CAD build for the part. Positions are in the model's coordinates, mm. Face numbers are marked on the shaded views. Round coordinates to 2 decimals unless told otherwise and drop trailing zeros. Loops run counter-clockwise (first coordinate to the right, second up) from the corner with the lowest first, then second, coordinate; pieces in that order, holes last. Notation, with made-up numbers: M 39,80 L 50,80 A17 cw 50,97 Z; hole C -34,-36.5 d10. An arc over 180 degrees is marked long. Put each result on its own line as item: value. Start each with the question number.
Autodesk Inventor part; units mm, degrees
ref_plane "YZ Plane" through (0, 0, 0) normal (1, 0, 0) x (0, 1, 0)
ref_plane "XZ Plane" through (0, 0, 0) normal (0, 1, 0) x (-1, 0, 0)
ref_plane "XY Plane" through (0, 0, 0) normal (0, 0, 1) x (1, 0, 0)
sketch "Sketch1" plane through (0, 0, 0) normal (0, 1, 0) x (-1, 0, 0)
  line L0 (0, 0) -> (0, -88.265)
  line L1 (0, -88.265) -> (41.275, -88.265)
  line L2 (0, 0) -> (23.8125, 0)
  line L3 (32.4358, -34.29) -> (32.4358, -59.69)
  line L4 (41.275, -88.265) -> (41.275, -81.915)
  line L5 (23.8125, 0) -> (23.8125, -6.35)
  line L6 (23.8125, -6.35) -> (32.4358, -34.29)
  line L7 (32.4358, -59.69) -> (41.275, -81.915)
  line L8 (33.655, -88.265) -> (33.655, -80.645)
  line L9 (7.62, -88.265) -> (7.62, -80.645)
  line L10 (7.62, -80.645) -> (33.655, -80.645)
  line L11 (16.1925, 0) -> (16.1925, -7.62)
  line L12 (16.1925, -7.62) -> (7.62, -7.62)
  line L13 (7.62, -7.62) -> (7.62, 0)
  point P0 (32.4358, -46.99)
  dimension "d0" = 88.265
  dimension "d1" = 41.275
  dimension "d2" = 23.8125
  dimension "d3" = 41.275
  dimension "d4" = 32.4358
  dimension "d5" = 25.4
  dimension "d6" = 12.7
  dimension "d10" = 6.35
  dimension "d11" = 6.35
  dimension "d12" = 7.62
  dimension "d13" = 7.62
  dimension "d14" = 7.62
  dimension "d15" = 7.62
  dimension "d16" = 7.62
  dimension "d17" = 7.62
extrude "Extrusion1" add sketch "Sketch1" along normal blind 6.985 contours L2 L13 L12 L11 L5 L6 L3 L7 L4 L1 L8 L10 L9 L0
fillet "Fillet2" radius 3.175 12 edges at (-41.275, 3.4925, -81.915) (-32.4358, 3.4925, -59.69) (-32.4358, 3.4925, -34.29) (-23.8125, 3.4925, -6.35) (-3.81, 0, 0) (-3.81, 6.985, 0) (-20.0025, 0, 0) (-20.0025, 6.985, 0) (-37.465, 0, -88.265) (-37.465, 6.985, -88.265) (-3.81, 0, -88.265) (-3.81, 6.985, -88.265)
sketch "Sketch2" plane through (0, 6.985, 0) normal (0, 1, 0) x (1, 0, 0)
  line L0 (-7.62, 85.09) -> (0, 85.09)
  line L1 (-7.62, 85.09) -> (-7.62, 80.645)
  line L2 (-7.62, 80.645) -> (-33.655, 80.645)
  line L3 (-33.655, 80.645) -> (-33.655, 85.09)
  line L4 (-41.275, 85.09) -> (-33.655, 85.09)
  line L5 (-41.275, 85.09) -> (-41.275, 82.5232)
  arc A0 (-41.275, 82.5232) -> (-41.0502, 81.3499) centre (-38.1, 82.5232) ccw
  line L6 (-41.0502, 81.3499) -> (-32.6606, 60.2551)
  arc A1 (-32.4358, 59.0818) -> (-32.6606, 60.2551) centre (-35.6108, 59.0818) ccw
  line L7 (-32.4358, 59.0818) -> (-32.4358, 34.7688)
  arc A2 (-32.4358, 34.7688) -> (-32.2946, 33.8325) centre (-29.2608, 34.7688) ccw
  line L8 (-32.2946, 33.8325) -> (-23.9537, 6.8075)
  arc A3 (-23.8125, 5.8712) -> (-23.9537, 6.8075) centre (-26.9875, 5.8712) ccw
  line L9 (-23.8125, 5.8712) -> (-23.8125, 3.175)
  line L10 (-16.1925, 3.175) -> (-23.8125, 3.175)
  line L11 (-16.1925, 3.175) -> (-16.1925, 7.62)
  line L12 (-16.1925, 7.62) -> (-7.62, 7.62)
  line L13 (-7.62, 7.62) -> (-7.62, 3.175)
  line L14 (0, 3.175) -> (-7.62, 3.175)
  line L15 (0, 3.175) -> (0, 85.09)
  line L16 (-22.9108, 35.7265) -> (-22.9108, 59.0818)
  arc A4 (-22.9108, 59.0818) -> (-23.8099, 63.7752) centre (-35.6108, 59.0818) ccw
  line L17 (-23.8099, 63.7752) -> (-26.731, 71.12)
  line L18 (-26.731, 71.12) -> (-9.525, 71.12)
  line L19 (-9.525, 71.12) -> (-9.525, 17.145)
  line L20 (-9.525, 17.145) -> (-17.1759, 17.145)
  line L21 (-17.1759, 17.145) -> (-22.9108, 35.7265)
  line L22 (-32.4358, 59.0818) -> (-32.4358, 34.7688)
  line L23 (-32.4358, 53.8188) -> (-29.2608, 53.8188)
  line L24 (-29.2608, 53.8188) -> (-29.2608, 34.7688)
  line L25 (-29.2608, 34.7688) -> (-32.4358, 34.7688)
  line L26 (-32.4358, 34.7688) -> (-32.4358, 59.0818)
  line L27 (-19.7358, 54.7765) -> (-19.7358, 35.7265)
  line L28 (-19.7358, 35.7265) -> (-22.9108, 35.7265)
  line L29 (-19.7358, 35.7265) -> (-20.8902, 29.1796)
  line L30 (-22.9108, 35.7265) -> (-22.9108, 54.7765)
  line L31 (-22.9108, 54.7765) -> (-19.7358, 54.7765)
  point P0 (0, 0)
  dimension "d19" = 9.525
  dimension "d25" = 3.175
  dimension "d26" = 3.175
  dimension "d28" = 80
  dimension "d44" = 19.05
  dimension "d45" = 19.05
  dimension "d46" = 19.05
extrude "Extrusion2" cut sketch "Sketch2" against normal blind 6.985 contours L16 L31 L27 L28 | L16 A4 L17 L18 L19 L20 L21 L29 L27 L31
sketch "Sketch3" plane through (0, 6.985, 0) normal (0, 1, 0) x (1, 0, 0)
  line L0 (-32.4358, 59.0818) -> (-32.4358, 34.7688)
  line L1 (-32.4358, 59.0818) -> (-29.2608, 59.0818)
  line L2 (-29.2608, 59.0818) -> (-29.2608, 34.7688)
  line L3 (-29.2608, 34.7688) -> (-32.4358, 34.7688)
  line L4 (-32.4358, 34.7688) -> (-32.4358, 59.0818)
  line L5 (-20.8902, 29.1796) -> (-17.1759, 17.145)
  line L6 (-23.4823, 59.0818) -> (-22.9108, 59.0818)
  line L7 (-22.9108, 59.0818) -> (-22.9108, 35.7265)
  line L8 (-22.9108, 35.7265) -> (-23.4823, 35.7265)
  line L9 (-23.4823, 35.7265) -> (-23.4823, 59.0818)
  point P0 (0, 0)
  dimension "d22" = 3.175
  dimension "d24" = 5.7785
sketch "Sketch4" plane through (0, 6.985, 0) normal (0, 1, 0) x (1, 0, 0)
  line L0 (-32.4358, 53.8188) -> (-29.2608, 53.8188)
  line L1 (-29.2608, 53.8188) -> (-29.2608, 34.7688)
  line L2 (-29.2608, 34.7688) -> (-32.4358, 34.7688)
  line L3 (-32.4358, 34.7688) -> (-32.4358, 53.8188)
  line L4 (-20.2438, 59.0818) -> (-20.2438, 35.7265)
  line L5 (-20.2438, 53.8188) -> (-23.4188, 53.8188)
  line L6 (-23.4188, 53.8188) -> (-23.4188, 35.7265)
  line L7 (-23.4188, 35.7265) -> (-20.2438, 35.7265)
  line L8 (-20.2438, 35.7265) -> (-20.2438, 59.0818)
  point P0 (0, 0)
  dimension "d29" = 3.175
  dimension "d30" = 3.175
  dimension "d43" = 19.05
extrude "Extrusion3" add sketch "Sketch4" against normal blind 17.78
sketch "Sketch5" plane through (-32.4358, 6.985, -59.0818) normal (-1, 0, 0) x (0, 0, 1)
  circle A0 centre (20.757, -14.732) radius 1.27
  line L0 (0, 0) -> (24.313, 0)
  circle A1 centre (14.5613, -12.446) radius 1.27
  circle A2 centre (8.3655, -10.16) radius 1.27
  line L1 (24.313, -6.985) -> (24.313, -17.78)
  line L2 (20.757, -14.732) -> (8.3655, -10.16) construction
  point P0 (59.0818, -6.985)
  dimension "d33" = 2.54
  dimension "d34" = 14.732
  dimension "d35" = 2.54
  dimension "d36" = 6.604
  dimension "d37" = 2.54
  dimension "d38" = 6.604
  dimension "d39" = 10.16
  dimension "d40" = 3.556
extrude "Extrusion4" cut sketch "Sketch5" against normal blind 25.4
sketch "Sketch6" plane through (-23.8125, 0, -5.8712) normal (-1, 0, 0) x (0, 0, 1)
  circle A0 centre (2.5695, 3.5161) radius 1.651
  point P0 (5.8712, 0)
  dimension "d47" = 3.302
equation "\"d38\" = d36"
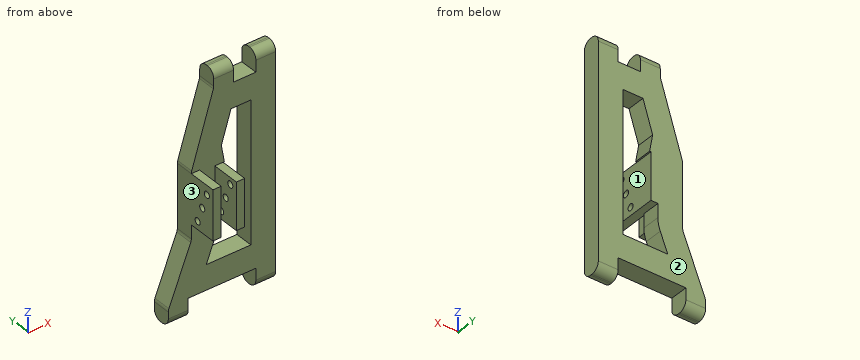
(1) Flat gauge pins, fed straight in: pin 1 Ø4 at (y, z) = (-3.18, -50.72) entering from +X; pin 2 Ø7.5 at (y, z) = (3, -3) entering from -X; pin 3 Ø4 at (y, z) = (-5.46, -44.52) entering from -X. Where does each tip first touch, or does it go through?
(2) Cut at C-C on x = -5.5. List the corners of the cut face in (y, z) (3 decimals), and give its area (3 significant figures).
(3) Cut at B-B on z = -19. List the corners of the cut face in (x, y) (3 decimals).
(4) Cut at D-D on z = -78. List the corners of the cut face in (x, y) (3 decimals), and give its area (3 significant figures).
(5) Drill centre lines: line 1 along X through (y, z) = (3.5, -45) (3 decimals); line 2 along Z through (x, y) = (-14, 4.25) (3 decimals); line 3 along Y through (x, z) = (-4, -8.5) (3 decimals). Where is each one in solid material? Low to high.
(6) Mould opens along X. For the marked faces 1, 2 and 3 say: +X half, -X half, draft (parallel to the pull), parting line (faces both ways), or undercut.
Taken from the geometry:
1. pin 1: x = -20.24
1. pin 2: x = -23.94
1. pin 3: x = -32.44
2. outline: M 0,-85.09 A3.175 ccw 3.175,-88.265 L 3.81,-88.265 A3.175 ccw 6.985,-85.09 L 6.985,-3.175 A3.175 ccw 3.81,0 L 3.175,0 A3.175 ccw 0,-3.175 Z
2. area: 608 mm2
3. outline: M -27.717,0 L -17.748,0 L -17.748,6.985 L -27.717,6.985 Z; M -9.525,0 L 0,0 L 0,6.985 L -9.525,6.985 Z
4. outline: M -39.718,0 L 0,0 L 0,6.985 L -39.718,6.985 Z
4. area: 277 mm2
5. line 1: -32.436 to -20.244, -9.525 to 0
5. line 2: -80.645 to -71.12, -17.145 to -7.62
5. line 3: 0 to 6.985
6. face 1: undercut
6. face 2: draft
6. face 3: -X half
